Design review of the part built by this model. Coordinates are the model's own, in mm. Face numbers are marked on the shaded views. Give positions to 0.01 mm unless a question says otherwise; leave off trailing zeros. Write each loop counter-clockwise with the first axis right and the second up, starting at its lowest first coordinate (ties: lowest second). Pieces come first, ordered by that corner, then holes. Notation, with made-up numbers: (-34, 1.5) -> (12, 1.5) arc R25 ccw to (12, 29.5) -> close; hole circle Ø11 at (-20, 35). An arc over 180 degrees is marked (long way). Write each question's results on one line, items separated by ' | '. Start each with the question number.
(1) To check wall thickness, follow probe 1 along Y at (x, z) = (0, 1.85); probe 2 along X at (y, z) = (0, 2.1); probe 3 along Y at (x, z) = (1.25, 1.35). State the ranges of each line that lie inside material, in increasing order.
(2) Take a section at C-C (z = 0.75). State the section outline as (x, y) points, plus the area to 3 significant figures.
(3) Take a section at A-A (x = -10.75). State the section outline as (y, z) points, plus the area to 3 significant figures.
(4) Clearance check with flat-ended pins moving along their axes: pin 1 (4.5 mm diameter, centred on x = -9.5, y = 0, fed in from +Z); pin 2 (1.5 mm diameter, centred on x = 2, z = 1, fed in from -Y); pin 3 (4 mm diameter, centred on x = 0, y = -8, fed in from +Z); pin 4 (1 mm diameter, centred on x = 9, y = 1, fed in from -Z). State where each tip first meets the part, or that it passes through.
(5) Mouldability with a two-part tool opening along Y and no side actions: class the marked faces 1, 2 and 3 as released by +Y, released by -Y, zero draft, split by the parting line, or undercut.
(6) Take a section at B-B (y = 0). State the section outline as (x, z) points.
(7) Take a section at D-D (x = 0). State the section outline as (y, z) points, plus the area to 3 significant figures.
from build123d import *

# Parameters (mm, degrees)
F0_R     = 14
F0_R_2   = 1.75
F0_R_3   = 5.1
F1_DEPTH = 10
F5_W     = 30
F5_H     = 3
F6_DEPTH = 40


with BuildPart() as f1:
    # F0 (on Top) → F1 (new body)
    with BuildSketch(Plane.XY):
        Circle(F0_R)
        with Locations((0, -8)):
            Circle(F0_R_2, mode=Mode.SUBTRACT)
        with Locations((-9.5, 0)):
            Circle(F0_R_2, mode=Mode.SUBTRACT)
        Circle(F0_R_3, mode=Mode.SUBTRACT)
        with Locations((9.5, 0)):
            Circle(F0_R_2, mode=Mode.SUBTRACT)
        with Locations((0, 8)):
            Circle(F0_R_2, mode=Mode.SUBTRACT)
    extrude(amount=F1_DEPTH)

    # F5 (on face) → F6 (intersect)
    with BuildSketch(Plane(origin=(17.6776695297, -17.6776695297, 0), x_dir=(0.7071067812, 0.7071067812, 0), z_dir=(0.7071067812, -0.7071067812, 0))):
        Polygon((-15, 5.6246599058), (-15, 0), (15, 0), (15, 3), align=None)
        with Locations((0, -1.5)):
            Rectangle(F5_W, F5_H)
    extrude(amount=-F6_DEPTH, mode=Mode.INTERSECT)


solid = f1.part
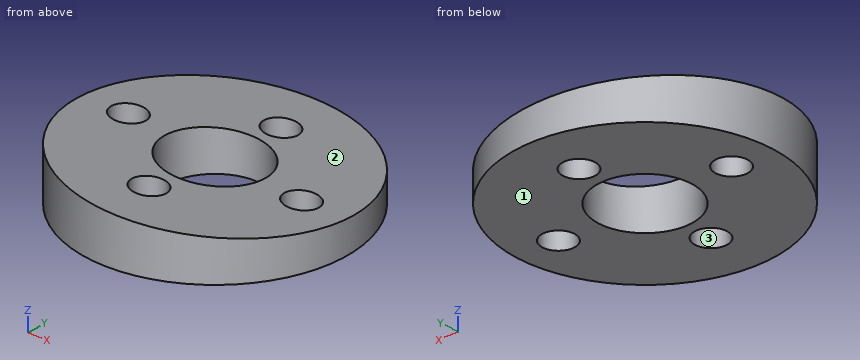
Report:
1) probe 1: -14 to -9.75, -6.25 to -5.1, 5.1 to 6.25, 9.75 to 14 | probe 2: -14 to -11.25, -7.75 to -5.1, 5.1 to 7.75, 11.25 to 14 | probe 3: -13.94 to -9.22, -6.78 to -4.94, 4.94 to 6.78, 9.22 to 13.94
2) outline: circle Ø28 at (0, 0); hole circle Ø3.5 at (-9.5, 0); hole circle Ø10.2 at (0, 0); hole circle Ø3.5 at (0, -8); hole circle Ø3.5 at (0, 8); hole circle Ø3.5 at (9.5, 0) | area: 496 mm2
3) outline: (-8.97, 0) -> (-1.22, 0) -> (-1.22, 5.05) -> (-8.97, 5.53) -> close; (1.22, 0) -> (8.97, 0) -> (8.97, 4.42) -> (1.22, 4.9) -> close | area: 77.1 mm2
4) pin 1: z = 5.1 | pin 2: y = -13.94 | pin 3: z = 4.98 | pin 4: through
5) face 1: zero draft | face 2: released by +Y | face 3: undercut
6) outline: (-14, 0) -> (-11.25, 0) -> (-11.25, 5.01) -> (-14, 5.18) -> close; (-7.75, 0) -> (-5.1, 0) -> (-5.1, 4.63) -> (-7.75, 4.79) -> close; (5.1, 0) -> (7.75, 0) -> (7.75, 3.83) -> (5.1, 4) -> close; (11.25, 0) -> (14, 0) -> (14, 3.45) -> (11.25, 3.62) -> close
7) outline: (-14, 0) -> (-9.75, 0) -> (-9.75, 4.92) -> (-14, 5.18) -> close; (-6.25, 0) -> (-5.1, 0) -> (-5.1, 4.63) -> (-6.25, 4.7) -> close; (5.1, 0) -> (6.25, 0) -> (6.25, 3.93) -> (5.1, 4) -> close; (9.75, 0) -> (14, 0) -> (14, 3.45) -> (9.75, 3.71) -> close | area: 46.6 mm2
